Part model, mm, in its own coordinate system. Round coordinates to 2 decimals unless told otherwise and drop trailing zeros. Write each loop counter-clockwise with the first axis right and the second up, starting at its lowest first coordinate (ties: lowest second). Pieces come first, ordered by that corner, then holes.
from build123d import *

# Parameters (mm, degrees)
SKETCH1_R           = 31.75
SKETCH1_R_2         = 1.90000001
BOSS_EXTRUDE1_DEPTH = 3.175


with BuildPart() as part:
    # Sketch1 → Boss-Extrude1 (new body, symmetric)
    with BuildSketch(Plane(origin=(0, 0, 0), x_dir=(1, 0, 0), z_dir=(0, 1, 0))):
        Circle(SKETCH1_R)
        with Locations((21.997045256, 12.7)):
            Circle(SKETCH1_R_2, mode=Mode.SUBTRACT)
        with Locations((21.997045256, -12.7)):
            Circle(SKETCH1_R_2, mode=Mode.SUBTRACT)
        with Locations((-12.7, -21.997045256)):
            Circle(SKETCH1_R_2, mode=Mode.SUBTRACT)
        with Locations((12.7, -21.997045256)):
            Circle(SKETCH1_R_2, mode=Mode.SUBTRACT)
        with Locations((-21.997045256, 12.7)):
            Circle(SKETCH1_R_2, mode=Mode.SUBTRACT)
        with Locations((-21.997045256, -12.7)):
            Circle(SKETCH1_R_2, mode=Mode.SUBTRACT)
        with Locations((12.7, 21.997045256)):
            Circle(SKETCH1_R_2, mode=Mode.SUBTRACT)
        with Locations((-12.7, 21.997045256)):
            Circle(SKETCH1_R_2, mode=Mode.SUBTRACT)
    extrude(amount=BOSS_EXTRUDE1_DEPTH, both=True)


solid = part.part
Q1. Drop flat-ended pins along their axis: P1, Ø3, axis at x = 22, z = -12.7, coming from the -Y side; P2, Ø2, axis at x = 14.5, y = 0, coming from the -Z side; P3, Ø1.5, axis at x = -14, y = -1, coming from the +Z side; P4, Ø4.5, axis at x = -22, z = 12.7, coming from the -Y side (3 decimals). Give the stop position or say it passes through.
Q2. Saw through at A-A, the plane x = -12.7. Write the cut outline in (y, z) (3 decimals).
Q3. Wall check: line 1 (Z direction, x = -22, y = 0); line 2 (X direction, y = 1.25, z = 12.7); line 3 (Z direction, x = 20.5, y = 0). Give the ranges that are in metal, low to high.
Q4. Saw through at C-C, the plane y = 1.5. Give the number of separate pieces and of enclosed holes in the cut face, and give its area (3 significant figures).
Q5. Two-plate mould, pull along Z, no slides. Class faces 1 (the cylindrical face through (-6.883, 0.044, 30.995)), 2 (the flat face through (0, 3.175, 0)), 3 (the cylindrical face through (-12.947, -0.044, 20.113)), 4 (the cylindrical face through (21.585, -0.044, -10.845)): released by +Z, released by -Z, zero draft, split by the parting line, or undercut.
Q6. Saw through at B-B, the plane z = 12.7. Write the cut outline in (x, y) (3 decimals).
Q7. Saw through at D-D, the plane x = -5.5. Write the cut outline in (y, z) (3 decimals).
Computed:
1. P1: passes through
1. P2: stops at z = -28.74
1. P3: stops at z = 28.85
1. P4: stops at y = -3.175
2. outline: (-3.175, -29.099) - (3.175, -29.099) - (3.175, -23.897) - (-3.175, -23.897) - close; (-3.175, -20.097) - (3.175, -20.097) - (3.175, 20.097) - (-3.175, 20.097) - close; (-3.175, 23.897) - (3.175, 23.897) - (3.175, 29.099) - (-3.175, 29.099) - close
3. line 1: z = -22.89 to -14.6, -10.8 to 10.8, 14.6 to 22.89
3. line 2: x = -29.1 to -23.9, -20.1 to 20.1, 23.9 to 29.1
3. line 3: z = -24.24 to -13.87, -11.53 to 11.53, 13.87 to 24.24
4. separate pieces: 1
4. enclosed holes: 8
4. area: 3,080 mm2
5. face 1: split by the parting line
5. face 2: zero draft
5. face 3: undercut
5. face 4: undercut
6. outline: (-29.099, -3.175) - (-23.897, -3.175) - (-23.897, 3.175) - (-29.099, 3.175) - close; (-20.097, -3.175) - (20.097, -3.175) - (20.097, 3.175) - (-20.097, 3.175) - close; (23.897, -3.175) - (29.099, -3.175) - (29.099, 3.175) - (23.897, 3.175) - close
7. outline: (-3.175, -31.27) - (3.175, -31.27) - (3.175, 31.27) - (-3.175, 31.27) - close
